Source: CAD feature listing. Evaluate the final solid. Frame: model axes, mm. A direction names the side the tool comes from. Give positions to 0.01 mm unless a question says otherwise; leave off trailing zeros. Order: outer loops, then holes, each group sorted by start corner. A loop starts at its lowest first (then second) coordinate and runs counter-clockwise, first axis right, second up. Notation, with made-up numbers: (38.25, -3) -> (97.25, -3) arc R6 ccw to (97.25, 6) -> close; hole circle Ø5 at (-1.5, -2). An arc over 180 degrees is marked (long way). Answer in a Markdown table with one row per item.
```python
from build123d import *

# Parameters (mm, degrees)
F1_DEPTH       = 19
F3_D           = 8.8
F3_CBORE_D     = 14.25
F3_CBORE_DEPTH = 2
F4_R           = 5
F6_D           = 8.8
F6_CBORE_D     = 14.25
F6_CBORE_DEPTH = 2
F7_R           = 5
F9_D           = 8.8


with BuildPart() as f1:
    # F0 (on Front) → F1 (new body)
    with BuildSketch(Plane.XZ):
        with BuildLine():
            ThreePointArc((-32.7130879295, 4.3421052632), (0, 33), (32.7130879295, 4.3421052632))
            ThreePointArc((32.7130879295, 4.3421052632), (34.3748837654, 1.2390510716), (37.6696164037, 0))
            Line((37.6696164037, 0), (70, 0))
            Line((70, 0), (70, 10))
            Line((70, 10), (50.8330601086, 10))
            ThreePointArc((50.8330601086, 10), (47.8393560232, 10.9952857968), (46.0374884002, 13.5849056604))
            ThreePointArc((46.0374884002, 13.5849056604), (43.5031680278, 20.2848310702), (40, 26.5329983228))
            Line((40, 26.5329983228), (40, 103))
            Line((40, 103), (0, 103))
            Line((0, 103), (-40, 103))
            Line((-40, 103), (-40, 26.5329983228))
            ThreePointArc((-40, 26.5329983228), (-43.5031680278, 20.2848310702), (-46.0374884002, 13.5849056604))
            ThreePointArc((-46.0374884002, 13.5849056604), (-47.8393560232, 10.9952857968), (-50.8330601086, 10))
            Line((-50.8330601086, 10), (-70, 10))
            Line((-70, 10), (-70, 0))
            Line((-70, 0), (-37.6696164037, 0))
            ThreePointArc((-37.6696164037, 0), (-34.3748837654, 1.2390510716), (-32.7130879295, 4.3421052632))
        make_face()
    extrude(amount=F1_DEPTH)

    # F3 (through all)
    with Locations(Plane.XY.offset(10)):
        with Locations((60.4165300543, -9.5)):
            CounterBoreHole(F3_D / 2, F3_CBORE_D / 2, F3_CBORE_DEPTH)

    # F4
    f4_edges = [f1.edges().sort_by_distance(p)[0] for p in [
        (70, -19, 5),
        (70, 0, 5),
    ]]
    fillet(f4_edges, radius=F4_R)

    # F6 (through all)
    with Locations(Plane.XY.offset(10)):
        with Locations((-60.4165300543, -9.5)):
            CounterBoreHole(F6_D / 2, F6_CBORE_D / 2, F6_CBORE_DEPTH)

    # F7
    f7_edges = [f1.edges().sort_by_distance(p)[0] for p in [
        (-70, -19, 5),
        (-70, 0, 5),
    ]]
    fillet(f7_edges, radius=F7_R)

    # F9 (through all)
    with Locations(Plane.XY.offset(103)):
        with Locations((20, -9.5), (-20, -9.5)):
            Hole(F9_D / 2)


solid = f1.part
```
(1) Ray query, probe 1 along X at (y, z) = (-11.5, 73); probe 2 along X at (y, z) = (-6, 57.5); probe 3 along Y at (x, z) = (-20, 56). Return the intervals inside material, ascending.
A:
| item | result |
|---|---|
| probe 1 | x = -40 to -23.92, -16.08 to 16.08, 23.92 to 40 |
| probe 2 | x = -40 to -22.67, -17.33 to 17.33, 22.67 to 40 |
| probe 3 | y = -19 to -13.9, -5.1 to 0 |
(2) Section query A-A (z = 35). Return the cut outline in (x, y), plus the area to 3 significant figures.
A:
| item | result |
|---|---|
| outline | (-40, -19) -> (40, -19) -> (40, 0) -> (-40, 0) -> close; hole circle Ø8.8 at (-20, -9.5); hole circle Ø8.8 at (20, -9.5) |
| area | 1,400 mm^2 |
(3) Access query for faces 1 (the cylindrical face through (34.34, -9.37, 1.27)), 2 (the flat face through (-54, -14, 10)), 3 (the flat face through (-1, 0, 52)), 4 (the cylindrical face through (67.213, -7.36, 9.014)), 5 (the flat face through (54, -14, 10)). Directions: +Z, -Z, +X, -X, +Y, -Y. A direction counts if a zero-diameter tool reaches every point of the face in a straight line with its end or side. Return the directions, or none.
A:
| item | result |
|---|---|
| face 1 | -Z, +Y, -Y |
| face 2 | +Z, -X, +Y, -Y |
| face 3 | +Z, -Z, +X, -X, +Y |
| face 4 | +Z |
| face 5 | +Z, +X, +Y, -Y |
(4) First-contact query: pin 1 Ø3 at (y, z) = (-10.5, 23) entering from +X; pin 2 Ø8 at (x, y) = (-16, -2.5) entering from -Z; pin 3 Ø9.5 at (y, z) = (-8, 50) entering from +X; pin 4 Ø3 at (x, z) = (12, 70) entering from +Y. Flat tips, straight axial feed; report the tip coordinate or a pass-through.
A:
| item | result |
|---|---|
| pin 1 | stops at x = 42.92 |
| pin 2 | stops at z = 26.25 |
| pin 3 | stops at x = 40 |
| pin 4 | stops at y = 0 |
(5) Section query D-D (x = 49). Return the cut outline in (y, z), plus the area to 3 significant figures.
A:
| item | result |
|---|---|
| outline | (-19, 0) -> (0, 0) -> (0, 10.35) -> (-19, 10.35) -> close |
| area | 197 mm^2 |
(6) Section query C-C (y = -11). Give the number of separate pieces and of enclosed holes in the cut face, plus the area to 3 significant figures.
A:
| item | result |
|---|---|
| separate pieces | 5 |
| enclosed holes | 0 |
| area | 5,800 mm^2 |
(7) Section query B-B (x = -22). Return the cut outline in (y, z).
A:
| item | result |
|---|---|
| outline | (-19, 24.6) -> (-13.42, 24.6) -> (-13.42, 103) -> (-19, 103) -> close; (-5.58, 24.6) -> (0, 24.6) -> (0, 103) -> (-5.58, 103) -> close |
